Input: part model. Units: mm. Frame: model coordinates. A direction names the side the tool comes from. Give positions to 0.01 mm unless a question says otherwise; leave off trailing zeros. Order: outer loops, then holes, each group sorted by start corner. A loop starts at its lowest first (then second) coordinate and runs counter-clockwise, first axis right, second up. Notation, with made-up numbers: M 67,-19.5 L 98,-19.5 A21 cw 98,4.5 Z; hole C -34,84 d9. An arc over 180 degrees is marked long. Use a Markdown table: item, result.
from build123d import *

# Parameters (mm, degrees)
SKETCH1_R             = 15
BOSS_EXTRUDE1_DEPTH   = 11
SKETCH2_R             = 3.175
CUT_EXTRUDE1_DEPTH    = 23
SKETCH3_R             = 17
CUT_EXTRUDE2_DEPTH    = 11
CUT_EXTRUDE3_DEPTH    = 11
SKETCH5_W             = 16.165630516
SKETCH5_H             = 1
CUT_EXTRUDE4_DEPTH    = 21
SKETCH6_R             = 2
CUT_EXTRUDE5_DEPTH    = 21
CUT_EXTRUDE6_START    = -4.2
SKETCH7_R             = 3.75
CUT_EXTRUDE6_DEPTH    = 21
M4_TAPPED_HOLE1_D     = 3.3
M4_TAPPED_HOLE1_DEPTH = 20.1
M4_TAPPED_HOLE1_TIP   = 0.991420021
CHAMFER2_SIZE         = 0.1
PAH1_SIZE             = 0.4
IZIM1_R               = 0.3


with BuildPart() as part:
    # Sketch1 → Boss-Extrude1 (new, symmetric)
    with BuildSketch(Plane(origin=(0, 0, 0), x_dir=(1, 0, 0), z_dir=(0, 1, 0))):
        with Locations(Location((0, 0, 0), (0, 0, 270))):
            Circle(SKETCH1_R)
    extrude(amount=BOSS_EXTRUDE1_DEPTH, both=True)

    # Sketch2 → Cut-Extrude1 (cut)
    with BuildSketch(Plane(origin=(0, 11, 0), x_dir=(1, 0, 0), z_dir=(0, 1, 0))):
        with Locations(Location((0, 0, 0), (0, 0, 270))):
            Circle(SKETCH2_R)
    extrude(amount=-CUT_EXTRUDE1_DEPTH, mode=Mode.SUBTRACT)

    # Sketch3 → Cut-Extrude2 (cut)
    with BuildSketch(Plane(origin=(0, 11, 0), x_dir=(1, 0, 0), z_dir=(0, 1, 0))):
        with Locations((16, 0)):
            Circle(SKETCH3_R)
    extrude(amount=-CUT_EXTRUDE2_DEPTH, mode=Mode.SUBTRACT)

    # Sketch4 → Cut-Extrude3 (cut)
    with BuildSketch(Plane(origin=(0, 11, 0), x_dir=(1, 0, 0), z_dir=(0, 1, 0))):
        with BuildLine():
            ThreePointArc((-6, 13.747727085), (-15, 0), (-6, -13.747727085))
            ThreePointArc((-6, -13.747727085), (-1.6187903, -9.065363068), (0.716230469, -3.093160021))
            ThreePointArc((0.716230469, -3.093160021), (-3.175, 0), (0.716230469, 3.093160021))
            ThreePointArc((0.716230469, 3.093160021), (-1.6187903, 9.065363068), (-6, 13.747727085))
        make_face()
    extrude(amount=-CUT_EXTRUDE3_DEPTH, mode=Mode.SUBTRACT)

    # Sketch5 → Cut-Extrude4 (cut)
    with BuildSketch(Plane(origin=(0, 0, 0), x_dir=(1, 0, 0), z_dir=(0, 1, 0))):
        with Locations((11.807437966, 0)):
            Rectangle(SKETCH5_W, SKETCH5_H)
    extrude(amount=-CUT_EXTRUDE4_DEPTH, mode=Mode.SUBTRACT)

    # Sketch6 → Cut-Extrude5 (cut)
    with BuildSketch(Plane.XY):
        with Locations(Location((11, -5.5, 0), (0, 0, 180))):
            Circle(SKETCH6_R)
    extrude(amount=CUT_EXTRUDE5_DEPTH, mode=Mode.SUBTRACT)

    # Sketch7 → Cut-Extrude6 (cut)
    with BuildSketch(Plane(origin=(0, 0, 0.5), x_dir=(-1, 0, 0), z_dir=(0, 0, -1)).offset(CUT_EXTRUDE6_START)):
        with Locations((-11, -5.5)):
            Circle(SKETCH7_R)
    extrude(amount=-CUT_EXTRUDE6_DEPTH, mode=Mode.SUBTRACT)

    # M4 Tapped Hole1
    with Locations(Plane.XY.offset(-0.5)):
        with Locations((11, -5.5)):
            Hole(M4_TAPPED_HOLE1_D / 2, depth=M4_TAPPED_HOLE1_DEPTH)
            with Locations((0, 0, -(M4_TAPPED_HOLE1_DEPTH + M4_TAPPED_HOLE1_TIP / 2))):  # 118° drill point
                Cone(0, M4_TAPPED_HOLE1_D / 2, M4_TAPPED_HOLE1_TIP, mode=Mode.SUBTRACT)

    # Chamfer2
    chamfer2_edges = [part.edges().sort_by_distance(p)[0] for p in [
        (-15, -11, 0),
    ]]
    chamfer(chamfer2_edges, length=CHAMFER2_SIZE)

    # Pah1
    pah1_edges = [part.edges().sort_by_distance(p)[0] for p in [
        (2.398064099, 11, -10.197418288),
        (2.398064099, 11, 10.197418288),
        (-2.398064099, 11, 10.197418288),
        (-2.398064099, 11, -10.197418288),
    ]]
    chamfer(pah1_edges, length=PAH1_SIZE)

    # Çizim1 → Kes-Döndür4 (revolve, cut)
    with BuildSketch(Plane(origin=(0, 0, 0), x_dir=(0, 0, -1), z_dir=(1, 0, 0))):
        with Locations((15, 0.05)):
            Circle(IZIM1_R)
    revolve(axis=Axis((0, -10.9, 0), (0, 1, 0)), mode=Mode.SUBTRACT)


solid = part.part
1) Reachability of faces 5 (the face through (9, -5, -0.5)), 6 (the face through (-3.5, 0, -0.2)), 7 (the face through (-2.27, 10.71, -10.21)), 8 (the face through (9, -7, 4.7)) from +Z, -Z, +X, -X, +Y, -Y: full face, straight path, thin tool, end or side. Return the list, or none.
Response values:
| item | result |
|---|---|
| face 5 | +X, +Y, -Y |
| face 6 | +Y |
| face 7 | -X, +Y |
| face 8 | +Z |
2) Cut plane D-D on z = 2. State how many separate pieces and enclosed holes the cut face has, and give its area (3 significant figures).
Response values:
| item | result |
|---|---|
| separate pieces | 2 |
| enclosed holes | 1 |
| area | 260 mm² |
3) First-contact query: pin 1 Ø5.5 at (x, y) = (7, -4.5) entering from +Z; pin 2 Ø5.5 at (x, y) = (11.5, -4) entering from +Z; pin 3 Ø9 at (x, y) = (10, -6.5) entering from -Z. Flat tips, straight axial feed; report the tip coordinate or a pass-through.
Response values:
| item | result |
|---|---|
| pin 1 | stops at z = 14.39 |
| pin 2 | stops at z = 11.54 |
| pin 3 | stops at z = -13.96 |
4) Cut plane B-B on y = 6.5. Return loops of the section in (x, z), and give its area (3 significant figures).
Response values:
| item | result |
|---|---|
| outline | M -6,-13.75 A15 ccw 6,-13.75 A17 cw 0,-5.74 A17 cw Z; M -6,13.75 A17 cw 0,5.74 A17 cw 6,13.75 A15 ccw Z |
| area | 96.1 mm² |
5) Material intervals for line 1 (Y direction, x = 11, z = 6); line 2 (Z direction, x = 0, y = -6.5) (3 decimals); line 3 (Y direction, x = 11, z = 2.5), sorted ascending. Write a range as from..to.
Response values:
| item | result |
|---|---|
| line 1 | y = -11..-9.25, -1.75..0 |
| line 2 | z = -15..-3.175, 3.175..15 |
| line 3 | y = -11..-7.5, -3.5..0 |
6) Mould query, pull axis Z, two halves, no side actions, for faces 1 (the face through (-14.986, -5.5, -0.653)), 2 (the face through (-2.44, 5.37, 10.25)), 3 (the face through (-3, -11, 3)), 4 (the face through (2.264, 10.714, 10.208)). Classes: released by +Z, released by -Z, zero draft, split by the parting line, or undercut.
Response values:
| item | result |
|---|---|
| face 1 | split by the parting line |
| face 2 | undercut |
| face 3 | zero draft |
| face 4 | undercut |
7) Cut plane C-C on y = -1. Return loops of the section in (x, z) (3 decimals).
Response values:
| item | result |
|---|---|
| outline | M 3.725,-0.5 L 3.725,0.5 L 14.992,0.5 A15 ccw long 14.992,-0.5 Z; hole C 0,0 d6.35 |
8) Cut plane A-A on y = -5.5. Return loops of the section in (x, z) (3 decimals), and give its area (3 significant figures).
Response values:
| item | result |
|---|---|
| outline | M 3.725,-0.5 L 3.725,0.5 L 9,0.5 L 9,4.7 L 7.25,4.7 L 7.25,13.132 A15 ccw long 9.35,-11.729 L 9.35,-0.5 Z; M 12.65,-8.061 A15 ccw 14.992,-0.5 L 12.65,-0.5 Z; M 13,0.5 L 14.992,0.5 A15 ccw 14.245,4.7 L 13,4.7 Z; hole C 0,0 d6.35 |
| area | 578 mm² |
